from build123d import *

# Parameters (mm, degrees)
BOSS_EXTRUDE1_DEPTH = 2
SKETCH2_R           = 2
CUT_EXTRUDE1_DEPTH  = 2
SKETCH3_R           = 2
CUT_EXTRUDE2_DEPTH  = 2


with BuildPart() as part:
    # Sketch1 → Boss-Extrude1 (new body)
    with BuildSketch(Plane.XY):
        Polygon((-41, 2), (-39, 0), (0, 0), (0, 20), (-30, 20), (-30, 28), (-32, 30), (-39, 30), (-41, 28), align=None)
        Polygon((0, 20), (0, 0), (39, 0), (41, 2), (41, 28), (39, 30), (32, 30), (30, 28), (30, 20), align=None)
    extrude(amount=BOSS_EXTRUDE1_DEPTH)

    # Sketch2 → Cut-Extrude1 (cut)
    with BuildSketch(Plane.XY.offset(2)):
        with Locations((-36, 24)):
            Circle(SKETCH2_R)
        with Locations((36, 24)):
            Circle(SKETCH2_R)
    extrude(amount=-CUT_EXTRUDE1_DEPTH, mode=Mode.SUBTRACT)

    # Sketch3 → Cut-Extrude2 (cut)
    with BuildSketch(Plane(origin=(0, 0, 0), x_dir=(-1, 0, 0), z_dir=(0, 0, -1))):
        with Locations((-35, 10)):
            Circle(SKETCH3_R)
        with Locations((35, 10)):
            Circle(SKETCH3_R)
    extrude(amount=-CUT_EXTRUDE2_DEPTH, mode=Mode.SUBTRACT)


solid = part.part
Work out the finished part from the listing and answer in its coordinate system (mm). A direction names the side the tool comes from. Give positions to 0.01 mm unless a question says otherwise; leave off trailing zeros. Order: outer loops, then holes, each group sorted by start corner. A loop starts at its lowest first (then second) coordinate and runs counter-clockwise, first axis right, second up. Notation, with made-up numbers: (84.25, -27.5) -> (90.25, -27.5) arc R30 ccw to (90.25, 9.5) -> close; hole circle Ø4 at (77.5, -35). An arc over 180 degrees is marked (long way). Answer as a JSON object with one key per item and string values. Group by question number.
1. Consider line 1 along Y through (x, z) = (36.5, 1.2); line 2 along Y through (x, z) = (35, 1.3); line 3 along X through (y, z) = (25.25, 0.8). Determine where each line is inside the solid, lowest interval first. Write a range as [from, to].
2. Section B-B on y = 24 is taken. Determine the outline of the cut face in (x, z).
3. A flat-ended cylindrical pin translates along its axis: pin 1 Ø2.5 at (x, y) = (-36, 24) entering from +Z. Find the tip coordinate at first contact, or state that the pin passes through.
4. The mould has two halves that part along X. Classify faces 3 (the cylindrical face through (-36.908, 10.601, 0.986)), 4 (the flat face through (-1, 12, 0)), 5 (the flat face through (40, 1, 1)): released by +X, released by -X, zero draft, split by the parting line, or undercut.
5. Section C-C on z = 0.5 is taken. Determine the outline of the cut face in (x, y), plus the area to 3 significant figures.
6. Section D-D on x = 35 is taken. Determine the outline of the cut face in (y, z), plus the area to 3 significant figures.
7. A tool of negligible diameter and unlimited length cuts with its end or side. For faces 1 (the flat face through (-40, 1, 1)), 2 (the flat face through (0, 20, 1)), from which of +Z, -Z, +X, -X, +Y, -Y can it reach the whole face along a straight path? Write none if from no direction.
8. Section A-A on y = 10 is taken. Determine the outline of the cut face in (x, z), plus the area to 3 significant figures.
Result sheet:
{
 "1": {"line 1": "y = [0, 8.68], [11.32, 22.06], [25.94, 30]", "line 2": "y = [0, 8], [12, 22.27], [25.73, 30]", "line 3": "x = [-41, -37.56], [-34.44, -30], [30, 34.44], [37.56, 41]"},
 "2": {"outline": "(-41, 0) -> (-38, 0) -> (-38, 2) -> (-41, 2) -> close; (-34, 0) -> (-30, 0) -> (-30, 2) -> (-34, 2) -> close; (30, 0) -> (34, 0) -> (34, 2) -> (30, 2) -> close; (38, 0) -> (41, 0) -> (41, 2) -> (38, 2) -> close"},
 "3": {"pin 1": "passes through"},
 "4": {"face 3": "undercut", "face 4": "zero draft", "face 5": "released by +X"},
 "5": {"outline": "(-41, 2) -> (-39, 0) -> (39, 0) -> (41, 2) -> (41, 28) -> (39, 30) -> (32, 30) -> (30, 28) -> (30, 20) -> (-30, 20) -> (-30, 28) -> (-32, 30) -> (-39, 30) -> (-41, 28) -> close; hole circle Ø4 at (-36, 24); hole circle Ø4 at (-35, 10); hole circle Ø4 at (35, 10); hole circle Ø4 at (36, 24)", "area": "1,800 mm^2"},
 "6": {"outline": "(0, 0) -> (8, 0) -> (8, 2) -> (0, 2) -> close; (12, 0) -> (22.27, 0) -> (22.27, 2) -> (12, 2) -> close; (25.73, 0) -> (30, 0) -> (30, 2) -> (25.73, 2) -> close", "area": "45.1 mm^2"},
 "7": {"face 1": "+Z, -Z, -X, -Y", "face 2": "+Z, -Z, +Y"},
 "8": {"outline": "(-41, 0) -> (-37, 0) -> (-37, 2) -> (-41, 2) -> close; (-33, 0) -> (33, 0) -> (33, 2) -> (-33, 2) -> close; (37, 0) -> (41, 0) -> (41, 2) -> (37, 2) -> close", "area": "148 mm^2"}
}
